Study the drawing (mm; zero at the part's minimum x, y, z) and answer. Coordinates: 2 decimals unless noted, no trailing zeros. Write each loop counter-clockwise with the first axis right and the second up, starting at its lowest first coordinate (ties: lowest second). Pieces come first, ordered by that corner, then holes. Notation, with made-up numbers: M 30.5,-6.75 L 65.5,-6.75 A31 cw 65.5,19.25 Z; hole C 62.25,9 d11. An arc over 180 degrees is marked long. Answer as a JSON object with one key per item and string values. Group by question number.
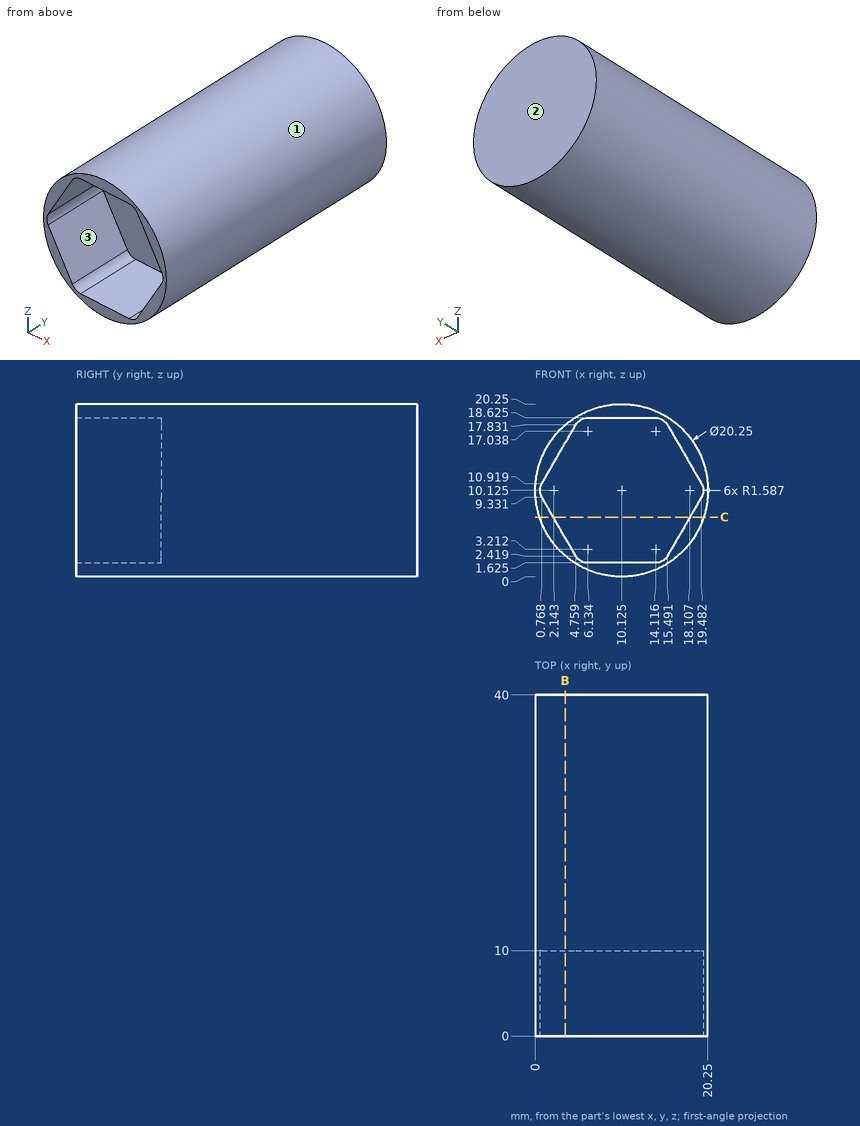
Item 1: For a pull along X with two mould halves and no side action, classify the marked faces 1, 2 and 3 as +X half, -X half, draft (parallel to the pull), parting line (faces both ways), or undercut.
Item 2: A cutting plane is placed at C-C, the plane z = 7. Write down the section's boundary in (x, y) (1 decimal), and give its area (3 significant figures).
Item 3: A cutting plane is placed at B-B, the plane x = 3.5. Write down the section's boundary in (y, z), and give its area (3 significant figures).
Item 4: Flat-ended cylindrical pins translate along their axes: pin 1 Ø1.5 at (x, y) = (6.5, 24) entering from +Z; pin 2 Ø1 at (x, y) = (4.5, 20.5) entering from +Z; pin 3 Ø4 at (x, y) = (3, 14.5) entering from -Z. Find the tip coordinate at first contact, or state that the pin passes through.
Item 5: Consider L1, parallel to Z at x = 10.5, y = 25; L2, parallel to Y at x = 3.25, z = 11.5; L3, parallel to X at y = 13, z = 14. Determine where each line is inside the solid, lowest interval first. Write a range as from..to.
Answer:
{
 "1": {"face 1": "parting line", "face 2": "draft", "face 3": "undercut"},
 "2": {"outline": "M 0.5,0 L 2.1,0 L 2.1,10 L 18.1,10 L 18.1,0 L 19.8,0 L 19.8,40 L 0.5,40 Z", "area": "610 mm2"},
 "3": {"outline": "M 0,2.47 L 40,2.47 L 40,17.78 L 0,17.78 L 0,15.65 L 10,15.65 L 10,4.6 L 0,4.6 Z", "area": "502 mm2"},
 "4": {"pin 1": "z = 19.83", "pin 2": "z = 18.86", "pin 3": "z = 1.39"},
 "5": {"L1": "0.01..20.24", "L2": "10..40", "L3": "0.77..19.48"}
}
